For this review, take the finished solid that the model builds, in its own axes (mm). A direction names the side the tool comes from. Give positions to 0.01 mm unless a question says otherwise; leave off trailing zeros. Order: outer loops, then holes, each group sorted by start corner. A loop starts at its lowest first (then second) coordinate and runs counter-clockwise, first axis right, second up. Notation, with made-up numbers: (-24, -36.5) - (28, -36.5) arc R22 cw to (28, -6.5) - close; hole circle Ø6 at (-21, 36.5). An arc over 180 degrees is marked (long way). Use a Markdown table: item, result. Add a question column.
1) We need section B-B on y = 6.5. Write out the cut boundary in (x, z).
2) Clearance check with flat-ended pins moving along their axes: P1, Ø1.5, axis at x = -1.5, z = -2, coming from the -Y side; P2, Ø1.5, axis at x = 0.5, z = 0.5, coming from the -Y side; P3, Ø1, axis at x = -2.5, y = 12, coming from the +Z side; P4, Ø3, axis at x = 1, z = -5, coming from the -Y side. State where each tip first meets the part, or that it passes through.
3) We need section D-D on z = 7.25. Write out the cut boundary in (x, y), then the cut area to 3 significant figures.
4) We need section C-C on z = 3.5. Write out the cut boundary in (x, y), then the cut area to 3 significant figures.
5) We need section A-A on x = 0. Write out the cut boundary in (y, z).
6) Machinability: for faces 1 (the face through (-0.54, -2.44, 8.48)), 2 (the face through (-1, 6, 1)), 3 (the face through (-2.5, -0.1, -5.1)), which of the approach directions +Z, -Z, +X, -X, +Y, -Y give a long, thin tool a straight path to every point of the face, cutting with its end or side? Answer none if there is none.
7) Wall thickness on L1, parallel to X at y = 10, z = 3.5; L2, parallel to X at y = 1, z = 3.5; L3, parallel to Z at x = 0, y = -0.5: over which ranges is each line inside the solid? List them lowest first.
```python
from build123d import *

# Parameters (mm, degrees)
EXTRUDE_1_DEPTH     = 7
SKETCH_3_R          = 2.5
EXTRUDE_2_DEPTH     = 3
EXTRUDE_START       = 10
SKETCH_4_R          = 2.5
EXTRUDE_3_DEPTH     = 10
SKETCH_5_R          = 2.5
SKETCH_5_R_2        = 1.5
EXTRUDE_5_DEPTH     = 8
SKETCH_6_R          = 1.5
CUT_EXTRUDE_6_DEPTH = 15.230249471


with BuildPart() as part:
    # 草圖1 → 伸長1 (new body)
    with BuildSketch(Plane.XY):
        with BuildLine():
            Line((-3.5, 0), (-3.5, 6))
            Line((-3.5, 6), (3.5, 6))
            Line((3.5, 6), (3.5, 0))
            ThreePointArc((3.5, 0), (0, -3.5), (-3.5, 0))
        make_face()
    extrude(amount=EXTRUDE_1_DEPTH)

    # 草圖3 → 伸長2 (add)
    with BuildSketch(Plane.XY.offset(7)):
        Circle(SKETCH_3_R)
    extrude(amount=EXTRUDE_2_DEPTH)

    # 草圖4 → 伸長3 (add)
    with BuildSketch(Plane(origin=(0, 0, 0), x_dir=(-1, 0, 0), z_dir=(0, 0, -1)).offset(EXTRUDE_START)):
        with Locations(Location((0, 0, 0), (0, 0, 180))):
            Circle(SKETCH_4_R)
    extrude(amount=-EXTRUDE_3_DEPTH)

    # 草圖5 → 伸長5 (add)
    with BuildSketch(Plane(origin=(0, 6, 0), x_dir=(1, 0, 0), z_dir=(0, 1, 0))):
        with Locations(Location((0, -3.5, 0), (0, 0, 90))):
            Circle(SKETCH_5_R)
        with Locations(Location((0, -3.5, 0), (0, 0, 270))):
            Circle(SKETCH_5_R_2, mode=Mode.SUBTRACT)
    extrude(amount=EXTRUDE_5_DEPTH)

    # 草圖6 → 伸長6 (cut, through all)
    with BuildSketch(Plane(origin=(0, 6, 0), x_dir=(1, 0, 0), z_dir=(0, 1, 0))):
        with Locations(Location((0, -3.5, 0), (0, 0, 270))):
            Circle(SKETCH_6_R)
    extrude(amount=-CUT_EXTRUDE_6_DEPTH, mode=Mode.SUBTRACT)


solid = part.part
```
Checked values:
| question | item | result |
|---|---|---|
| 1 | outline | circle Ø5 at (0, 3.5); hole circle Ø3 at (0, 3.5) |
| 2 | P1 | y = -2.38 |
| 2 | P2 | y = -3.5 |
| 2 | P3 | z = 5 |
| 2 | P4 | y = -2.5 |
| 3 | outline | circle Ø5 at (0, 0) |
| 3 | area | 19.6 mm² |
| 4 | outline | (-3.5, 0) arc R3.5 ccw to (-1.5, -3.16) - (-1.5, 14) - (-2.5, 14) - (-2.5, 6) - (-3.5, 6) - close; (1.5, -3.16) arc R3.5 ccw to (3.5, 0) - (3.5, 6) - (2.5, 6) - (2.5, 14) - (1.5, 14) - close |
| 4 | area | 49.1 mm² |
| 5 | outline | (-3.5, 0) - (-2.5, 0) - (-2.5, -10) - (2.5, -10) - (2.5, 0) - (6, 0) - (6, 1) - (14, 1) - (14, 2) - (-3.5, 2) - close; (-3.5, 5) - (14, 5) - (14, 6) - (6, 6) - (6, 7) - (2.5, 7) - (2.5, 10) - (-2.5, 10) - (-2.5, 7) - (-3.5, 7) - close |
| 6 | face 1 | +Z |
| 6 | face 2 | +Y |
| 6 | face 3 | -Z |
| 7 | L1 | -2.5 to -1.5, 1.5 to 2.5 |
| 7 | L2 | -3.5 to -1.5, 1.5 to 3.5 |
| 7 | L3 | -10 to 2, 5 to 10 |
